```python
from build123d import *

# Parameters (mm, degrees)
F0_W     = 290
F0_H     = 150
F1_DEPTH = 12
F2_R     = 15
F4_D     = 8.5
F3_W     = 115
F3_H     = 8
F5_DEPTH = 1
F6_D     = 6.8


with BuildPart() as f1:
    # F0 (on Top) → F1 (new body)
    with BuildSketch(Plane.XY):
        with Locations((0, 75)):
            Rectangle(F0_W, F0_H)
    extrude(amount=-F1_DEPTH)

    # F2
    f2_edges = [f1.edges().sort_by_distance(p)[0] for p in [
        (-145, 150, -6),
        (-145, 0, -6),
        (145, 150, -6),
        (145, 0, -6),
    ]]
    fillet(f2_edges, radius=F2_R)

    # F4 (through all)
    with Locations(Plane.XY):
        with Locations((130, 135), (130, 15), (-130, 135), (-130, 15)):
            Hole(F4_D / 2)

    # F3 (on face) → F5 (cut)
    with BuildSketch(Plane.XY):
        with Locations((0, -4)):
            Rectangle(F3_W, F3_H)
        with BuildLine():
            Line((57.5, 0), (57.5, 30))
            ThreePointArc((57.5, 30), (51.6421356237, 44.1421356237), (37.5, 50))
            Line((37.5, 50), (-37.5, 50))
            ThreePointArc((-37.5, 50), (-51.6421356237, 44.1421356237), (-57.5, 30))
            Line((-57.5, 30), (-57.5, 0))
            Line((-57.5, 0), (57.5, 0))
        make_face()
    extrude(amount=-F5_DEPTH, mode=Mode.SUBTRACT)

    # F6 (through all)
    with Locations(Plane.XY):
        with Locations((38, 22), (-38, 22)):
            Hole(F6_D / 2)


solid = f1.part
```
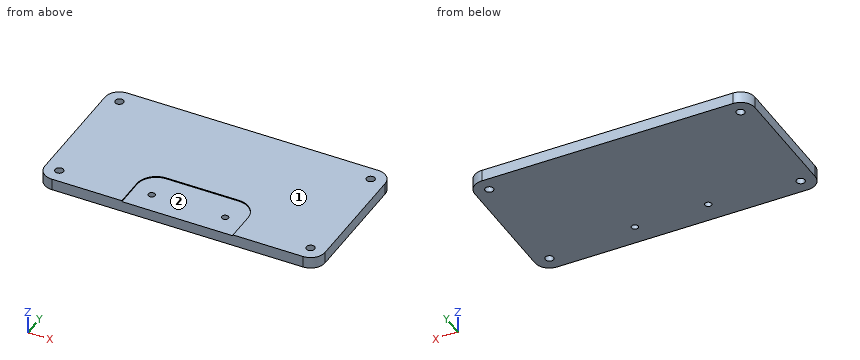
Can you work these out from the model? Positions are in its coordinate system, mm. Face numbers are marked on the shaded views. Coordinates: 2 decimals unless noted, no trailing zeros. Loops run counter-clockwise (first coordinate to the right, second up) from the corner with the lowest first, then second, coordinate; pieces in that order, holes last.
Item 1: If we mould it in two halves opening along X, with no side actions, what happens to the marked faces 1 and 2? For each: released by +X, released by -X, zero draft, split by the parting line, or undercut.
Answers below:
face 1: zero draft
face 2: undercut
Item 2: Suppose I cut it at A-A (y = 22). Please give me the cut outline in (x, z), then the cut area to 3 significant figures.
Answers below:
outline: (-145, -12) - (-41.4, -12) - (-41.4, -1) - (-57.5, -1) - (-57.5, 0) - (-145, 0) - close; (-34.6, -12) - (34.6, -12) - (34.6, -1) - (-34.6, -1) - close; (41.4, -12) - (145, -12) - (145, 0) - (57.5, 0) - (57.5, -1) - (41.4, -1) - close
area: 3,220 mm2
Item 3: I'm going to push flat-ended pins straight in: pin 1 (7.5 mm diameter, centred on x = 130, y = 15, fed in from -Z); pin 2 (1.1 mm diameter, centred on y = 12, z = -0.5, fed in from +X); pin 3 (15 mm diameter, centred on x = 24, y = 27, fed in from +Z). Where does each tip first touch, or does it pass through?
Answers below:
pin 1: passes through
pin 2: stops at x = 144.8
pin 3: stops at z = -1
Item 4: Please list where these lines run through material, in increasing order: L1, parallel to Y at x = -130, z = -4; L2, parallel to Y at x = 38, z = -3.75; L3, parallel to X at y = 138, z = -1.25.
Answers below:
L1: y = 0 to 10.75, 19.25 to 130.75, 139.25 to 150
L2: y = 0 to 18.6, 25.4 to 150
L3: x = -144.7 to -133.01, -126.99 to 126.99, 133.01 to 144.7
Item 5: Suppose I cut it at B-B (x = -22.5). Please give me the cut outline in (y, z).
Answers below:
outline: (0, -12) - (150, -12) - (150, 0) - (50, 0) - (50, -1) - (0, -1) - close
